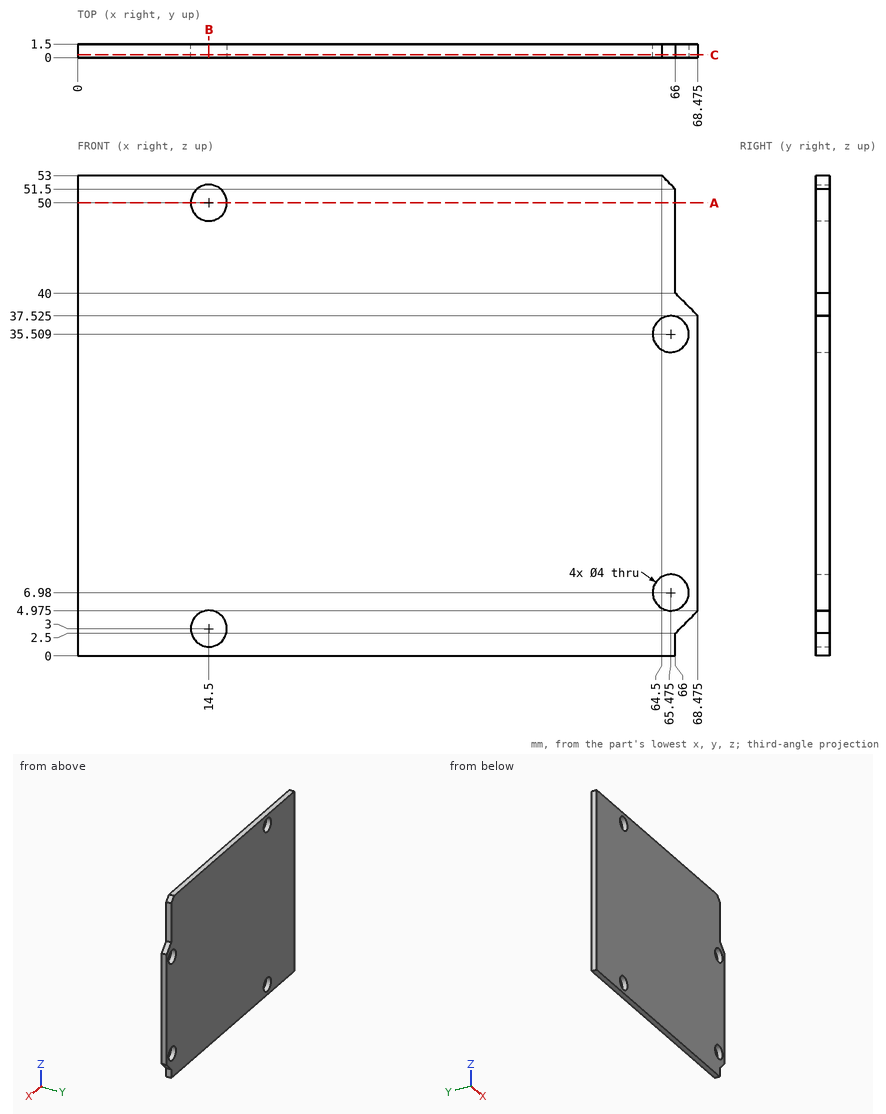
Drawing for the job (mm, zero at the part's lowest x, y, z). Round coordinates to 2 decimals unless told otherwise and drop trailing zeros. Write each loop counter-clockwise with the first axis right and the second up, starting at its lowest first coordinate (ties: lowest second). Pieces come first, ordered by that corner, then holes. Notation, with made-up numbers: (-24.5, -27.75) - (0.5, -27.75) arc R13 ccw to (0.5, -17.75) - close; hole circle Ø9 at (37.25, 13). An arc over 180 degrees is marked (long way). Write item = value, one per line. Start each with the question number.
Q1. Drop a flat-ended pin along its axis: pin 1 (3 mm diameter, centred on x = 14.5, z = 50, fed in from -Y). Give the stop position or say it passes through.
Q2. Band-saw the part on A-A (z = 50). Give the cut face in (x, y).
Q3. Probe L1, parallel to Z at x = 14.5, y = 1.15; L2, parallel to X at y = 0.9, z = 35.5 (1 decimal); L3, parallel to X at y = 1.4, z = 8.5 (1 decimal). List the from-to ranges inside material, lowest first. Write a range as from..to.
Q4. Band-saw the part on B-B (x = 14.5). Give the cut face in (y, z).
Q5. Band-saw the part on C-C (y = 0.3). Give the cut face in (x, z) (1 decimal), then the cut area to 3 significant figures.
Answers below:
q1.pin_1 = through
q2.outline = (0, 0) - (12.5, 0) - (12.5, 1.5) - (0, 1.5) - close; (16.5, 0) - (66, 0) - (66, 1.5) - (16.5, 1.5) - close
q3.L1 = 0..1, 5..48, 52..53
q3.L2 = 0..63.5, 67.5..68.5
q3.L3 = 0..64.2, 66.8..68.5
q4.outline = (0, 0) - (1.5, 0) - (1.5, 1) - (0, 1) - close; (0, 5) - (1.5, 5) - (1.5, 48) - (0, 48) - close; (0, 52) - (1.5, 52) - (1.5, 53) - (0, 53) - close
q5.outline = (0, 0) - (66, 0) - (66, 2.5) - (68.5, 5) - (68.5, 37.5) - (66, 40) - (66, 51.5) - (64.5, 53) - (0, 53) - close; hole circle Ø4 at (14.5, 3); hole circle Ø4 at (14.5, 50); hole circle Ø4 at (65.5, 7); hole circle Ø4 at (65.5, 35.5)
q5.area = 3,530 mm2
